```python
from build123d import *

# Parameters (mm, degrees)
SKETCH_1_R      = 1.5
EXTRUDE_1_DEPTH = 3
FILLET_1_R      = 20


with BuildPart() as part:
    # 草图1 → 凸台-拉伸1 (new body)
    with BuildSketch(Plane.XY):
        Polygon((0, 108.239220029), (-76.536686473, 76.536686473), (-108.239220029, 0), (-76.536686473, -76.536686473), (0, -108.239220029), (76.536686473, -76.536686473), (108.239220029, 0), (76.536686473, 76.536686473), align=None)
        with Locations((-46.741505227, -16.11378879)):
            Circle(SKETCH_1_R, mode=Mode.SUBTRACT)
        with Locations((-16.892197502, -88.176392326)):
            Circle(SKETCH_1_R, mode=Mode.SUBTRACT)
        with Locations((74.294712357, -50.405537551)):
            Circle(SKETCH_1_R, mode=Mode.SUBTRACT)
        with Locations((44.445404632, 21.657065985)):
            Circle(SKETCH_1_R, mode=Mode.SUBTRACT)
    extrude(amount=EXTRUDE_1_DEPTH)

    # 圆角1
    fillet_1_edges = [part.edges().sort_by_distance(p)[0] for p in [
        (76.536686473, 76.536686473, 1.5),
        (108.239220029, 0, 1.5),
        (76.536686473, -76.536686473, 1.5),
        (0, -108.239220029, 1.5),
        (-76.536686473, -76.536686473, 1.5),
        (-108.239220029, 0, 1.5),
        (-76.536686473, 76.536686473, 1.5),
        (0, 108.239220029, 1.5),
    ]]
    fillet(fillet_1_edges, radius=FILLET_1_R)


solid = part.part
```
For this review, take the finished solid that the model builds, in its own axes (mm). Round coordinates to 2 decimals unless told otherwise and drop trailing zeros. Loops run counter-clockwise (first coordinate to the right, second up) from the corner with the lowest first, then second, coordinate; pieces in that order, holes last.
(1) We need section B-B (y = -29). Give the boundary of the cut face in (x, z), plus the area to 3 significant figures.
Returned:
outline: (-96.23, 0) - (96.23, 0) - (96.23, 3) - (-96.23, 3) - close
area: 577 mm2
(2) We need section C-C (x = -12.5). Give the boundary of the cut face in (y, z).
Returned:
outline: (-103.06, 0) - (103.06, 0) - (103.06, 3) - (-103.06, 3) - close
(3) Wall thickness on line 1 along Y through (x, z) = (-1, 0.65); line 2 along X through (y, z) = (-51, 1.3); line 3 along X through (y, z) = (-49.5, 0.75): over which ranges is each line inside the solid? List them lowest first.
Returned:
line 1: y = -106.57 to 106.57
line 2: x = -87.11 to 72.92, 75.67 to 87.11
line 3: x = -87.74 to 73.1, 75.49 to 87.74
(4) We need section A-A (z = 1.7). Give the boundary of the cut face in (x, y), plus the area to 3 significant figures.
Returned:
outline: (-105.07, -7.65) - (-79.71, -68.88) arc R20 ccw to (-68.88, -79.71) - (-7.65, -105.07) arc R20 ccw to (7.65, -105.07) - (68.88, -79.71) arc R20 ccw to (79.71, -68.88) - (105.07, -7.65) arc R20 ccw to (105.07, 7.65) - (79.71, 68.88) arc R20 ccw to (68.88, 79.71) - (7.65, 105.07) arc R20 ccw to (-7.65, 105.07) - (-68.88, 79.71) arc R20 ccw to (-79.71, 68.88) - (-105.07, 7.65) arc R20 ccw to start; hole circle Ø3 at (-46.74, -16.11); hole circle Ø3 at (-16.89, -88.18); hole circle Ø3 at (44.45, 21.66); hole circle Ø3 at (74.29, -50.41)
area: 33,000 mm2
(5) Clearance check with flat-ended pins moving along their axes: P1, Ø2.5, axis at x = -16.89, y = -88.18, coming from the -Z side; P2, Ø1.5, axis at y = -26, z = 2, coming from the -X side; P3, Ø1, axis at x = 22.5, z = 2.5, coming from the +Y side. State where each tip first meets the part, or that it passes through.
Returned:
P1: passes through
P2: stops at x = -97.78
P3: stops at y = 99.13
